Autodesk Inventor part; units mm, degrees
ref_plane "YZ Plane" through (0, 0, 0) normal (1, 0, 0) x (0, 1, 0)
ref_plane "XZ Plane" through (0, 0, 0) normal (0, 1, 0) x (-1, 0, 0)
ref_plane "XY Plane" through (0, 0, 0) normal (0, 0, 1) x (1, 0, 0)
sketch "Sketch1" plane through (0, 0, 0) normal (0, 0, 1) x (1, 0, 0)
  point P0 (0, 0)
sketch "Sketch2" plane through (0, 0, 0) normal (0, 0, 1) x (1, 0, 0)
  circle A0 centre (0, 0) radius 9.975
  circle A1 centre (0, 0) radius 3
  dimension "d0" = 19.95
  dimension "d1" = 6
extrude "Extrusion1" add sketch "Sketch2" along normal blind 3.5
sketch "Sketch3" plane through (0, 0, 3.5) normal (0, 0, 1) x (1, 0, 0)
  circle A0 centre (0, 0) radius 9
  dimension "d9" = 18
extrude "Extrusion2" add sketch "Sketch3" along normal blind 1
sketch "Sketch4" plane through (0, 0, 4.5) normal (0, 0, 1) x (1, 0, 0)
  circle A0 centre (0, 0) radius 5.5
  dimension "nozzleInner" = 11
extrude "Extrusion3" add sketch "Sketch4" along normal blind 2.25
chamfer "Chamfer1" distance 0.8 angle 45 1 edges at (-9, 0, 3.5)
sketch "Sketch5" plane through (0, 0, 6.75) normal (0, 0, 1) x (1, 0, 0)
  circle A0 centre (0, 0) radius 7.5
  dimension "d24" = 15
extrude "Extrusion4" add sketch "Sketch5" along normal blind 1.5
ref_plane "Work Plane2" through (0, 0, 23.25) normal (0, 0, 1) x (1, 0, 0)
sketch "Sketch8" plane through (0, 0, 23.25) normal (0, 0, 1) x (1, 0, 0)
  circle A0 centre (0, 0) radius 0.5
  circle A1 centre (0, 0) radius 0.75
  dimension "d39" = 1
  dimension "d40" = 1.5
extrude "Extrusion7" add sketch "Sketch8" against normal blind 15
draft "FaceDraft1" angle 7 pull direction (0, 0, 1) faces at (0.7476, -0.0603, 13.25) fixed edges at (-0.75, 0, 23.25)
chamfer "Chamfer2" distance 0.4 angle 45 5 edges at (-7.5, 0, 6.75) (-7.5, 0, 8.25) (-5.5, 0, 4.5) (-5.5, 0, 6.75) (-2.5918, 0, 8.25)
equation "\"d1\" = di"
equation "\"d4\" = d10"
equation "\"nozzleInner\" = 0.5 * dO"
equation "\"d39\" = iTip"
equation "\"d40\" = oTip"
equation "\"iTip\" = 1"
equation "\"oTip\" = 1.5"
properties part number "nozzle-tip1-0402" material "Steel, Mild"
Could you check a few things on this model? Use its own coordinates, in mm. A direction names the side the tool comes from. Give positions to 0.01 mm unless a question says otherwise; leave off trailing zeros. Order: outer loops, then holes, each group sorted by start corner. A loop starts at its lowest first (then second) coordinate and runs counter-clockwise, first axis right, second up.
Item 1: I need wall thicknesses on line 1 (Y direction, x = 0, z = 2.2) (3 decimals); line 2 (Z direction, x = 3.75, y = 6); line 3 (Z direction, x = -4, y = 0.75). Which ranges of each line are inside material? Lowest first, please.
Item 2: If we section it at A-A, the plane z = 17.5: Write out the boundary of the cut face in (x, y).
Item 3: If we section it at B-B, the plane z = 21.25: Write out the boundary of the cut face in (x, y).
Item 4: If we mould it in two halves opening along Z, with no side actions, what happens to faces 1 (the face through (0, 0, 3.5)), 2 (the face through (9.514, -2.996, 1.726)), 3 (the face through (1, 6, 6.75))? For each: pulls with the +Z half, pulls with the -Z half, needs draft (parallel to the pull), parting line crosses it, or undercut.
Item 5: I'm going to push flat-ended pins straight in: pin 1 (5.5 mm diameter, centred on x = 0, y = 0, fed in from -Z); pin 2 (4 mm diameter, centred on y = -2.5, z = 19, fed in from -X); pin 3 (1.5 mm diameter, centred on x = -2, y = -5, fed in from -Z); pin 4 (2 mm diameter, centred on x = -6, y = 4, fed in from +Z). Where does each tip first touch, or does it pass through?
Item 6: For faces 4 (the face through (-1.19, 5.37, 5.61)), 5 (the face through (1, -3, 8.25)), which set-ups out of +Z, -Z, +X, -X, +Y, -Y let a thin tool reach every point of the face, with its end or its side?
Values:
1. line 1: y = -9.975 to -3, 3 to 9.975
1. line 2: z = 0 to 4.5, 6.75 to 8.25
1. line 3: z = 0 to 8.25
2. outline: circle Ø2.91 at (0, 0); hole circle Ø1 at (0, 0)
3. outline: circle Ø1.99 at (0, 0); hole circle Ø1 at (0, 0)
4. face 1: pulls with the -Z half
4. face 2: needs draft
4. face 3: undercut
5. pin 1: stops at z = 3.5
5. pin 2: stops at x = -1.21
5. pin 3: stops at z = 0
5. pin 4: stops at z = 8.25
6. face 4: none
6. face 5: +Z
